```python
from build123d import *

# Parameters (mm, degrees)
F1_DEPTH = 29
F3_DEPTH = 38.001
F4_DEPTH = 11
F5_R     = 5


with BuildPart() as f1:
    # F0 (on Front) → F1 (new body, symmetric)
    with BuildSketch(Plane.XZ):
        with BuildLine():
            Line((-52.5, 0), (0, 0))
            Line((0, 0), (52.5, 0))
            Line((52.5, 0), (52.5, 9))
            Line((52.5, 9), (63.5, 9))
            ThreePointArc((63.5, 9), (55.006097, 29.506097), (34.5, 38))
            Line((34.5, 38), (0, 38))
            Line((0, 38), (-34.5, 38))
            ThreePointArc((-34.5, 38), (-55.006097, 29.506097), (-63.5, 9))
            Line((-63.5, 9), (-52.5, 9))
            Line((-52.5, 9), (-52.5, 0))
        make_face()
    extrude(amount=F1_DEPTH, both=True)

    # F2 (on face) → F3 (cut, through all)
    with BuildSketch(Plane.XY.offset(38)):
        with BuildLine():
            Line((-19.5, 4), (-34.5, 4))
            Line((-34.5, 4), (-34.5, -4))
            Line((-34.5, -4), (-19.5, -4))
            ThreePointArc((-19.5, -4), (-15.5, 0), (-19.5, 4))
        make_face()
        with BuildLine():
            Line((-34.5, -4), (-34.5, 4))
            Line((-34.5, 4), (-38.5, 4))
            ThreePointArc((-38.5, 4), (-42.5, 0), (-38.5, -4))
            Line((-38.5, -4), (-34.5, -4))
        make_face()
        with BuildLine():
            Line((34.5, -4), (34.5, 4))
            Line((34.5, 4), (19.5, 4))
            ThreePointArc((19.5, 4), (15.5, 0), (19.5, -4))
            Line((19.5, -4), (34.5, -4))
        make_face()
        with BuildLine():
            Line((38.5, 4), (34.5, 4))
            Line((34.5, 4), (34.5, -4))
            Line((34.5, -4), (38.5, -4))
            ThreePointArc((38.5, -4), (42.5, 0), (38.5, 4))
        make_face()
    extrude(amount=-F3_DEPTH, mode=Mode.SUBTRACT)

    # F2 (on face) → F4 (cut)
    with BuildSketch(Plane.XY.offset(38)):
        with BuildLine():
            Line((-34.5, 4), (-34.5, 18))
            Line((-34.5, 18), (-67.5, 18))
            Line((-67.5, 18), (-67.5, -18))
            Line((-67.5, -18), (-34.5, -18))
            Line((-34.5, -18), (-34.5, -4))
            Line((-34.5, -4), (-38.5, -4))
            ThreePointArc((-38.5, -4), (-42.5, 0), (-38.5, 4))
            Line((-38.5, 4), (-34.5, 4))
        make_face()
        with BuildLine():
            Line((34.5, 18), (-34.5, 18))
            Line((-34.5, 18), (-34.5, 4))
            Line((-34.5, 4), (-19.5, 4))
            ThreePointArc((-19.5, 4), (-15.5, 0), (-19.5, -4))
            Line((-19.5, -4), (-34.5, -4))
            Line((-34.5, -4), (-34.5, -18))
            Line((-34.5, -18), (34.5, -18))
            Line((34.5, -18), (34.5, -4))
            Line((34.5, -4), (19.5, -4))
            ThreePointArc((19.5, -4), (15.5, 0), (19.5, 4))
            Line((19.5, 4), (34.5, 4))
            Line((34.5, 4), (34.5, 18))
        make_face()
        with BuildLine():
            Line((74.5, 18), (34.5, 18))
            Line((34.5, 18), (34.5, 4))
            Line((34.5, 4), (38.5, 4))
            ThreePointArc((38.5, 4), (42.5, 0), (38.5, -4))
            Line((38.5, -4), (34.5, -4))
            Line((34.5, -4), (34.5, -18))
            Line((34.5, -18), (74.5, -18))
            Line((74.5, -18), (74.5, 18))
        make_face()
    extrude(amount=-F4_DEPTH, mode=Mode.SUBTRACT)

    # F5
    f5_edges = [f1.edges().sort_by_distance(p)[0] for p in [
        (0, -29, 38),
        (0, 29, 38),
    ]]
    fillet(f5_edges, radius=F5_R)


solid = f1.part
```
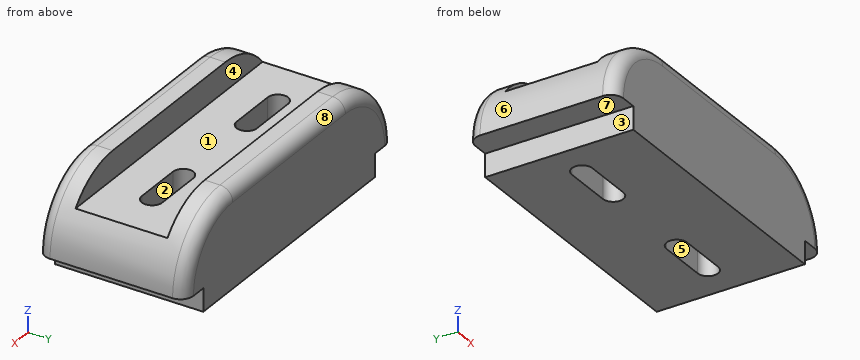
Can you work these out from the model? Positions are in its coordinate system, mm. Face numbers are marked on the shaded views. A direction names the side the tool comes from. Give positions to 0.01 mm unless a question says otherwise; leave off trailing zeros. Write each loop counter-clockwise with the first axis right and the second up, starting at its lowest first coordinate (ties: lowest second). Pieces come first, ordered by that corner, then holes. Notation, with made-up numbers: (-3.5, 25.25) -> (46.5, 25.25) arc R23 cw to (46.5, 36.25) -> close; hole circle Ø4 at (18, 24.5). An arc over 180 degrees is marked (long way). One line per item, written item: value.
Q1. Imagine slicing it at A-A on y = 0. Please give me the cut outline in (x, z).
Results found:
outline: (-63.5, 9) -> (-52.5, 9) -> (-52.5, 0) -> (-42.5, 0) -> (-42.5, 27) -> (-57.24, 27) arc R29 ccw to start; (-15.5, 0) -> (15.5, 0) -> (15.5, 27) -> (-15.5, 27) -> close; (42.5, 0) -> (52.5, 0) -> (52.5, 9) -> (63.5, 9) arc R29 ccw to (57.24, 27) -> (42.5, 27) -> close
Q2. Please list where these lines run through material, in increasing order: line 1 (Y direction, x = -28.5, z = 3.5); line 2 (Y direction, x = -20, z = 30); line 3 (Z direction, x = 55, y = -6.5). Write a range as [from, to].
Results found:
line 1: y = [-29, -4], [4, 29]
line 2: y = [-29, -18], [18, 29]
line 3: z = [9, 27]
Q3. Which directions (+Z, -Z, +X, -X, +Y, -Y) give clear straight access to the entire face, cutting with the end or side of a thin tool? Please do the marked faces 4, 5, 6, 7 and 8.
Results found:
face 4: +Z, +X, -X
face 5: +Z, -Z
face 6: +Z, -X, +Y, -Y
face 7: -Z, -X, +Y, -Y
face 8: +Z, +X, -X, +Y
Q4. Imagine slicing it at D-D on z = 24.5. Give the number of separate pieces and of enclosed holes in the cut face, and give its area (3 significant figures).
Results found:
separate pieces: 1
enclosed holes: 2
area: 6,410 mm^2
Q5. For P1, Ø12, axis at x = -57.5, y = -5.5, coming from the -Z side; P2, Ø5, axis at x = 42.5, y = 10, coming from the +Z side; P3, Ø3.5, axis at x = 58.5, y = 14.5, coming from the -Z side; P4, Ø4.5, axis at y = -8, z = 3.5, coming from the +X side, each with a flat end and sliding along its axis, tell me the tip position at first contact or that it passes through.
Results found:
P1: stops at z = 0
P2: stops at z = 27
P3: stops at z = 9
P4: stops at x = 52.5
Q6. We'd pull the mould along X, two halves only. Please class the marked faces 1, 2 and 3: +X half, -X half, draft (parallel to the pull), parting line (faces both ways), or undercut.
Results found:
face 1: draft
face 2: undercut
face 3: -X half
Q7. Imagine slicing it at B-B on x = -30.5. Please give me the cut outline in (y, z), and give its area (3 significant figures).
Results found:
outline: (-29, 0) -> (-4, 0) -> (-4, 27) -> (-18, 27) -> (-18, 38) -> (-24, 38) arc R5 ccw to (-29, 33) -> close; (4, 0) -> (29, 0) -> (29, 33) arc R5 ccw to (24, 38) -> (18, 38) -> (18, 27) -> (4, 27) -> close
area: 1,580 mm^2
Q8. Imagine slicing it at C-C on y = 13. Please give me the cut outline in (x, z).
Results found:
outline: (-63.5, 9) -> (-52.5, 9) -> (-52.5, 0) -> (52.5, 0) -> (52.5, 9) -> (63.5, 9) arc R29 ccw to (57.24, 27) -> (-57.24, 27) arc R29 ccw to start
